```python
from build123d import *

# Parameters (mm, degrees)
S01_TENDON_CAPTIVE_TAIL_R                      = 0.6
F_01_TENDON_CAPTIVE_TAIL_DEPTH                 = 12
S02_CROSSED_TENDON_R                           = 0.6
F_02_CROSSED_TENDON_DEPTH                      = 33.010681761
S03_TENDON_THROUGH_REAR_GROMMET_R              = 0.6
F_03_TENDON_THROUGH_REAR_GROMMET_DEPTH         = 12
F_04_START                                     = -0.55
F_04_TENDON_RETURN_DEPTH                       = 1.1
F_05_START                                     = 0.55
F_05_REMOVABLE_BACKED_EYE_AROUND_POLISHE_DEPTH = 1.1
S06_DRESSED_EYE_KNOT_ENVELOPE_R                = 2
F_06_DRESSED_EYE_KNOT_ENVELOPE_DEPTH           = 8.5


with BuildPart() as part:
    # S01 - Tendon captive tail → 01 - Tendon captive tail (new body)
    with BuildSketch(Plane.XY.offset(25.959868809)):
        with Locations((-14.854021031, 2.087596514)):
            Circle(S01_TENDON_CAPTIVE_TAIL_R)
    extrude(amount=F_01_TENDON_CAPTIVE_TAIL_DEPTH)

    # S02 - Crossed tendon → 02 - Crossed tendon (add)
    with BuildSketch(Plane(origin=(-5.56891097, -8.552306823, -12.992860813), x_dir=(0.9414814256928209, -0.18532252929363746, -0.28154623991739347), z_dir=(0.33706486775606503, 0.5176384007444039, 0.7864081389452696))):
        with Locations(Location((-21.680567016, -12.529320029, 0), (0, 0, 152.8840726))):
            Circle(S02_CROSSED_TENDON_R)
    extrude(amount=F_02_CROSSED_TENDON_DEPTH)

    # S03 - Tendon through rear grommet → 03 - Tendon through rear grommet (add)
    with BuildSketch(Plane.XY.offset(-12)):
        with Locations(Location((-25.980762114, -15, 0), (0, 0, 146.929477468))):
            Circle(S03_TENDON_THROUGH_REAR_GROMMET_R)
    extrude(amount=F_03_TENDON_THROUGH_REAR_GROMMET_DEPTH)

    # S04 - Tendon return → 04 - Tendon return (add)
    with BuildSketch(Plane(origin=(0, 0, 0), x_dir=(-0.8660254037844386, -0.5000000000000001, 0), z_dir=(0.5000000000000001, -0.8660254037844386, 0)).offset(F_04_START)):
        with BuildLine():
            Line((30.6, 12), (30.6, 45))
            ThreePointArc((30.6, 45), (27.788225099, 51.788225099), (21, 54.6))
            Line((21, 54.6), (-67.598500564, 54.6))
            Line((-67.598500564, 54.6), (-67.598500564, 53.4))
            Line((-67.598500564, 53.4), (21, 53.4))
            ThreePointArc((21, 53.4), (26.939696962, 50.939696962), (29.4, 45))
            Line((29.4, 45), (29.4, 12))
            Line((29.4, 12), (30.6, 12))
        make_face()
    extrude(amount=F_04_TENDON_RETURN_DEPTH)

    # S05 - Removable backed eye around polished clevis sleeve → 05 - Removable backed eye around polished clevis sleeve (add)
    with BuildSketch(Plane.XY.offset(-54).offset(F_05_START)):
        with BuildLine():
            Line((58.093813666, 34.175564254), (58.267018746, 34.275564254))
            ThreePointArc((58.267018746, 34.275564254), (63.936024172, 32.756558829), (62.417018746, 27.087553403))
            Line((62.417018746, 27.087553403), (52.890739305, 21.587553403))
            Line((52.890739305, 21.587553403), (46.269586882, 21.055725804))
            Line((46.269586882, 21.055725804), (40.755485267, 22.606429959))
            Line((40.755485267, 22.606429959), (41.221510671, 23.799250282))
            Line((41.221510671, 23.799250282), (46.562407205, 22.148546127))
            Line((46.562407205, 22.148546127), (52.817053277, 22.815181347))
            Line((52.817053277, 22.815181347), (61.867018746, 28.040181347))
            ThreePointArc((61.867018746, 28.040181347), (62.983396228, 32.206558829), (58.817018746, 33.32293631))
            Line((58.817018746, 33.32293631), (58.643813666, 33.22293631))
            Line((58.643813666, 33.22293631), (58.093813666, 34.175564254))
        make_face()
    extrude(amount=-F_05_REMOVABLE_BACKED_EYE_AROUND_POLISHE_DEPTH)

    # S06 - Dressed eye knot envelope → 06 - Dressed eye knot envelope (add)
    with BuildSketch(Plane(origin=(38.623434459, 22.299250282, 0), x_dir=(0, 0, -1), z_dir=(0.8660254037844386, 0.5000000000000001, 0))):
        with Locations(Location((54, 0, 0), (0, 0, 90))):
            Circle(S06_DRESSED_EYE_KNOT_ENVELOPE_R)
    extrude(amount=F_06_DRESSED_EYE_KNOT_ENVELOPE_DEPTH)


solid = part.part
```
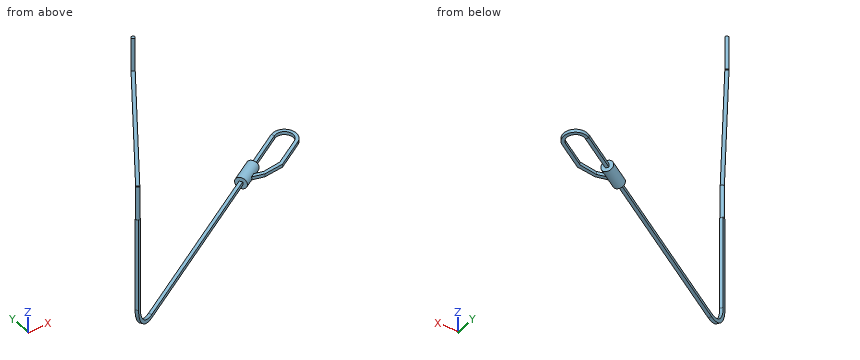
Verification items for the finished model (mm, model axes). Round coordinates to 2 decimals unless told otherwise and drop trailing zeros. Order: outer loops, then holes, each group sorted by start corner. A loop starts at its lowest first (then second) coordinate and runs counter-clockwise, first axis right, second up.
1) Material ranges on line 1 (Z direction, x = 40.5, y = 22); line 2 (Z direction, x = 40, y = 25), recorded low to high.
Geometry says:
line 1: z = -55.6 to -52.4
line 2: z = -55.13 to -52.87
2) Cross-section at A-A, the plane z = -19.5. Record the cut outline in (x, y).
Geometry says:
outline: (-26.78, -14.82) - (-26.23, -15.78) - (-25.19, -15.18) - (-25.74, -14.22) - close
3) Cross-section at B-B, the plane x = -4. Record the cut outline in (y, z).
Geometry says:
outline: (-2.94, -54.6) - (-1.67, -54.6) - (-1.67, -53.4) - (-2.94, -53.4) - close
4) Depth check by flat-ended pin: pin 1 (9 mm diameter, centred on x = 55.5, y = 30.5, fed in from +Z); pin 2 (4 mm diameter, centred on x = 51, y = 25, fed in from +Z); pin 3 (0.7 mm diameter, centred on x = -14.5, y = 2, fed in from -Z); pin 4 (6.5 mm diameter, centred on x = 52.5, y = 32, fed in from -Z). Enter the tip coordinate at first touch or a pass-through.
Geometry says:
pin 1: stops at z = -53.4
pin 2: passes through
pin 3: stops at z = 24.79
pin 4: stops at z = -54.6
